Drawing for the job (mm, zero at the part's lowest x, y, z). A direction names the side the tool comes from. Give positions to 0.01 mm unless a question says otherwise; leave off trailing zeros. Write each loop counter-clockwise with the first axis right and the second up, starting at its lowest first coordinate (ties: lowest second). Pieces come first, ordered by that corner, then holes.
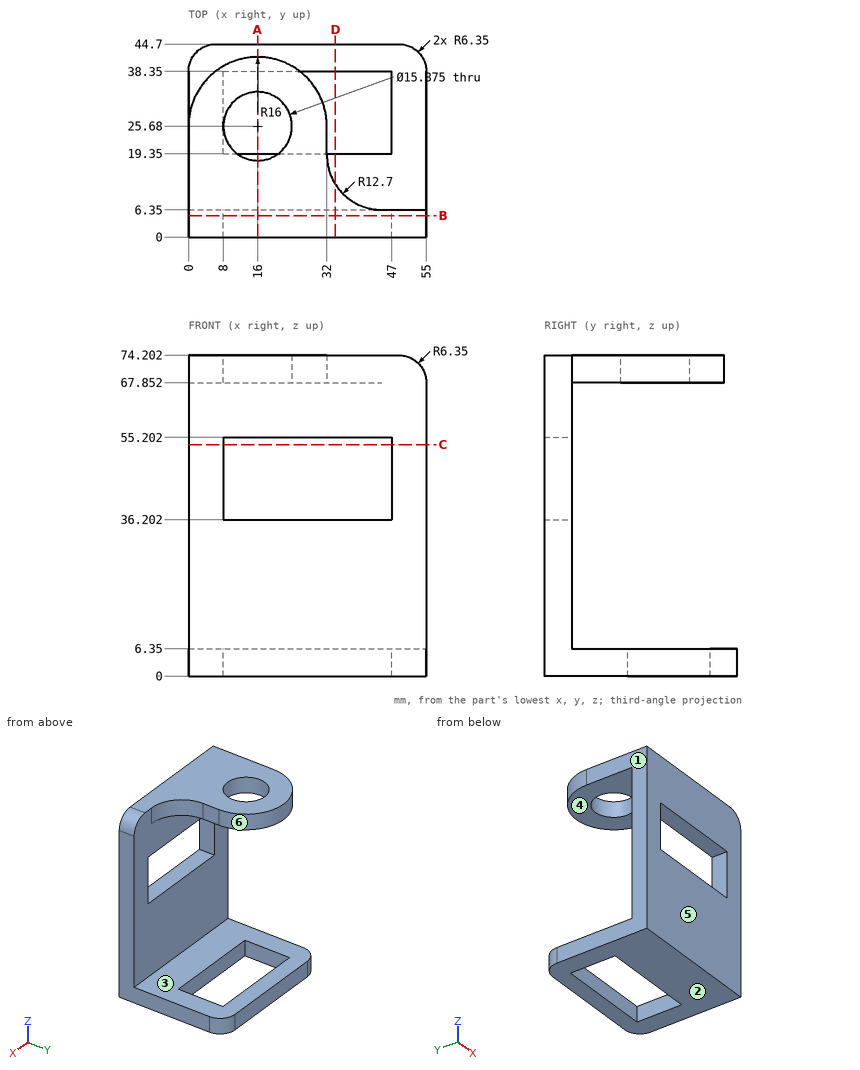
1. Slice it at A-A, the plane x = 16. Write the cut outline in (y, z), and give its area (3 significant figures).
Calculated:
outline: (0, 0) - (19.35, 0) - (19.35, 6.35) - (6.35, 6.35) - (6.35, 36.2) - (0, 36.2) - close; (0, 55.2) - (6.35, 55.2) - (6.35, 67.85) - (17.74, 67.85) - (17.74, 74.2) - (0, 74.2) - close; (33.62, 67.85) - (41.68, 67.85) - (41.68, 74.2) - (33.62, 74.2) - close; (38.35, 0) - (44.7, 0) - (44.7, 6.35) - (38.35, 6.35) - close
area: 597 mm2
2. Probe probe 1 along Y at (x, z) = (16, 71); probe 2 along X at (y, z) = (4, 47); probe 3 along Z at (x, y) = (7.5, 25). List the from-to ranges inside material, lowest first.
Calculated:
probe 1: y = 0 to 17.74, 33.62 to 41.68
probe 2: x = 0 to 8, 47 to 55
probe 3: z = 0 to 6.35, 67.85 to 74.2
3. Pin check, flat tips, straight feed: P1, Ø6, axis at x = 33.5, z = 34.5, coming from the +Y side; P2, Ø1, axis at y = 31, z = 8.5, coming from the +X side; P3, Ø1.9, axis at y = 22.5, z = 70, coming from the +X side. Stop position of each tip, or through.
Calculated:
P1: stops at y = 6.35
P2: passes through
P3: stops at x = 32
4. Slice it at C-C, the plane z = 53.5. Write the cut outline in (x, y).
Calculated:
outline: (0, 0) - (8, 0) - (8, 6.35) - (0, 6.35) - close; (47, 0) - (55, 0) - (55, 6.35) - (47, 6.35) - close
5. Which spindle directions (+Z, -Z, +X, -X, +Y, -Y) get a long thin tool onto all of the face, cutting with end or side? Do the marked faces 4, 5 and 6. Say none if no direction does.
Calculated:
face 4: +X, -X, +Y
face 5: +Z, -Z, +X, -X, -Y
face 6: +Z, +Y
6. Slice it at B-B, the plane y = 5. Write the cut outline in (x, z), and give its area (3 significant figures).
Calculated:
outline: (0, 0) - (55, 0) - (55, 67.85) arc R6.35 ccw to (48.65, 74.2) - (0, 74.2) - close; hole (8, 36.2) - (47, 36.2) - (47, 55.2) - (8, 55.2) - close
area: 3,330 mm2
7. Slice it at D-D, the plane x = 34. Write the cut outline in (y, z), and give its area (3 significant figures).
Calculated:
outline: (0, 0) - (19.35, 0) - (19.35, 6.35) - (6.35, 6.35) - (6.35, 36.2) - (0, 36.2) - close; (0, 55.2) - (6.35, 55.2) - (6.35, 67.85) - (12.21, 67.85) - (12.21, 74.2) - (0, 74.2) - close; (38.35, 0) - (44.7, 0) - (44.7, 6.35) - (38.35, 6.35) - close
area: 511 mm2
8. Pull direction Z, two halves, no side cores. Call the marked faces 1, 2 and 3: +Z half, -Z half, draft (parallel to the pull), parting line (faces both ways), or undercut.
Calculated:
face 1: draft
face 2: -Z half
face 3: undercut
